Work out the finished part from the listing and answer in its coordinate system (mm). A direction names the side the tool comes from. Round coordinates to 2 decimals unless told otherwise and drop trailing zeros. Write each loop counter-clockwise with the first axis right and the second up, starting at its lowest first coordinate (ties: lowest second). Pieces come first, ordered by that corner, then holes. Notation, with made-up numbers: M 47.25,-28 L 83.25,-28 A26 ccw 83.25,-12 Z; hole C 51,10.25 d11. An arc over 180 degrees is marked long. Answer in a Markdown table with one row per item.
```python
from build123d import *

# Parameters (mm, degrees)
F0_W      = 91.4067700505
F0_H      = 67.4502924085
F1_DEPTH  = 12.7
F3_DEPTH  = 25.4
F4_W      = 51.4017706737
F4_H      = 34.0803191066
F5_DEPTH  = 7.62
F6_W      = 21.1654342711
F6_H      = 34.0803191066
F7_DEPTH  = 25.4
F8_W      = 23.9177821204
F8_H      = 19.4233638573
F9_DEPTH  = 25.4
F10_W     = 14.652994927
F10_H     = 34.0803191066
F11_DEPTH = 7.62
F13_DEPTH = 10.16
F15_DEPTH = 25.4
F17_DEPTH = 25.4
F18_DEPTH = 10.16
F19_W     = 15.5833414756
F19_H     = 10.1625369862
F20_DEPTH = 10.16
F23_D     = 8.89


with BuildPart() as f1:
    # F0 (on Top) → F1 (new body)
    with BuildSketch(Plane.XY):
        with Locations((-3.4888088703, -14.8855820298)):
            Rectangle(F0_W, F0_H)
    extrude(amount=F1_DEPTH)

    # F2 (on face) → F3 (cut)
    with BuildSketch(Plane.XY.offset(12.7)):
        Polygon((-49.1921938956, 18.8395641744), (-49.1921938956, 0), (-15.6996361911, 18.8395641744), align=None)
        Polygon((-15.6996361911, -48.6107282341), (-49.1921938956, -23.0261329561), (-49.1921938956, -48.6107282341), align=None)
    extrude(amount=-F3_DEPTH, mode=Mode.SUBTRACT)

    # F4 (on face) → F5 (join)
    with BuildSketch(Plane.XY.offset(12.7)):
        with Locations((16.5136908181, -17.0401595533)):
            Rectangle(F4_W, F4_H)
    extrude(amount=F5_DEPTH)

    # F6 (on face) → F7 (join)
    with BuildSketch(Plane.XY.offset(20.32)):
        with Locations((31.6318590194, -17.0401595533)):
            Rectangle(F6_W, F6_H)
    extrude(amount=F7_DEPTH)

    # F8 (on face) → F9 (cut)
    with BuildSketch(Plane(origin=(21.0491418839, 0, 0), x_dir=(0, -1, 0), z_dir=(-1, 0, 0))):
        with Locations((22.1214280464, 30.0316819286)):
            Rectangle(F8_W, F8_H)
    extrude(amount=-F9_DEPTH, mode=Mode.SUBTRACT)

    # F10 (on face) → F11 (cut)
    with BuildSketch(Plane.XY.offset(20.32)):
        with Locations((-1.8606970552, -17.0401595533)):
            Rectangle(F10_W, F10_H)
    extrude(amount=-F11_DEPTH, mode=Mode.SUBTRACT)

    # F12 (on face) → F13 (join)
    with BuildSketch(Plane.XY.offset(20.32)):
        Polygon((21.0491418839, 0), (5.4658004083, 0), (5.4658004083, -13.4125072509), (21.0491418839, -13.4125072509), (21.0491418839, -10.1625369862), align=None)
    extrude(amount=F13_DEPTH)

    # F14 (on face) → F15 (cut)
    with BuildSketch(Plane.XY.offset(12.7)):
        Polygon((-28.525055022, -38.8135323032), (-28.525055022, 11.6252659037), (-49.1921938956, 0), (-49.1921938956, -23.0261329561), align=None)
    extrude(amount=-F15_DEPTH, mode=Mode.SUBTRACT)

    # F16 (on face) → F17 (cut)
    with BuildSketch(Plane.XY.offset(12.7)):
        Polygon((-28.525055022, 11.6252659037), (-28.525055022, -3.0236337334), (0, 18.8395641744), (-15.6996361911, 18.8395641744), align=None)
        Polygon((0, -48.6107282341), (-28.525055022, -28.1430520117), (-28.525055022, -38.8135323032), (-15.6996361911, -48.6107282341), align=None)
    extrude(amount=-F17_DEPTH, mode=Mode.SUBTRACT)

    # F18 (cut): a face of the model
    f18_faces = [f1.faces().sort_by_distance(p)[0] for p in [
        (13.2574711461, -6.7062536255, 30.48),
    ]]
    extrude(f18_faces, amount=-F18_DEPTH, mode=Mode.SUBTRACT)

    # F19 (on face) → F20 (join)
    with BuildSketch(Plane.XY.offset(20.32)):
        with Locations((13.2574711461, -5.0812684931)):
            Rectangle(F19_W, F19_H)
    extrude(amount=F20_DEPTH)

    # F23 (through all)
    with Locations(Plane.XY.offset(12.7)):
        with Locations((26.8638245761, 10.2338371798), (29.4222831726, -41.6331104934)):
            Hole(F23_D / 2)


solid = f1.part
```
1. Given pin 1 (1 mm diameter, centred on x = 24, z = 16, fed in from -Y); pin 2 (9 mm diameter, centred on y = -17, z = 25.5, fed in from -X); pin 3 (3 mm diameter, centred on x = 18, z = 23.5, fed in from +Y); pin 4 (10 mm diameter, centred on x = 26.86, y = 10.23, fed in from +Z), each flat-ended and moving along its own axis, determine where each tip first touches the part or whether it passes through.
Calculated:
| item | result |
|---|---|
| pin 1 | stops at y = -34.08 |
| pin 2 | passes through |
| pin 3 | stops at y = 0 |
| pin 4 | stops at z = 12.7 |
2. Determine the mould class of faces 1 (the flat face through (42.215, -15, 17)), 2 (the flat face through (24, -22, 20.32)), 3 (the flat face through (13, -5, 30.48)), 4 (the flat face through (28, -10.163, 28)) for opening direction Z: released by +Z, released by -Z, zero draft, split by the parting line, or undercut.
Calculated:
| item | result |
|---|---|
| face 1 | zero draft |
| face 2 | undercut |
| face 3 | released by +Z |
| face 4 | undercut |
3. A tool of negligible diameter and unlimited length cuts with its end or side. For faces 5 (the flat face through (24, -34.08, 16)), 6 (the flat face through (28, 0, 25)), 7 (the flat face through (31, -22, 39.743)), 8 (the flat face through (5.466, -13, 19)), from which of +Z, -Z, +X, -X, +Y, -Y can it reach the whole face along a straight path? Write none if from no direction.
Calculated:
| item | result |
|---|---|
| face 5 | +Z, +X, -X, -Y |
| face 6 | +Z, +X, -X, +Y |
| face 7 | +X, -X, -Y |
| face 8 | +Z, -X, +Y, -Y |
4. The part is cut by section B-B (x = 33). Determine the outline of the cut face in (y, z).
Calculated:
| item | result |
|---|---|
| outline | M -48.61,0 L -44.27,0 L -44.27,12.7 L -48.61,12.7 Z; M -39,0 L 18.84,0 L 18.84,12.7 L 0,12.7 L 0,45.72 L -34.08,45.72 L -34.08,39.74 L -10.16,39.74 L -10.16,20.32 L -34.08,20.32 L -34.08,12.7 L -39,12.7 Z |
5. Consider line 1 along Z through (x, y) = (32.5, -34); line 2 along X through (y, z) = (-6.5, 19.5); line 3 along Y through (x, z) = (9, 18.5). Determine where each line is inside the solid, lowest interval first. Write a range as from..to.
Calculated:
| item | result |
|---|---|
| line 1 | z = 0..20.32, 39.74..45.72 |
| line 2 | x = 5.47..42.21 |
| line 3 | y = -34.08..0 |
6. The part is cut by section A-A (y = -24). Determine the outline of the cut face in (x, z), plus the area to 3 significant figures.
Calculated:
| item | result |
|---|---|
| outline | M -28.53,0 L 42.21,0 L 42.21,20.32 L 5.47,20.32 L 5.47,12.7 L -28.53,12.7 Z; M 21.05,39.74 L 42.21,39.74 L 42.21,45.72 L 21.05,45.72 Z |
| area | 1,300 mm² |
7. The part is cut by section D-D (y = -8.5). Determine the outline of the cut face in (x, z).
Calculated:
| item | result |
|---|---|
| outline | M -28.53,0 L 42.21,0 L 42.21,45.72 L 21.05,45.72 L 21.05,30.48 L 5.47,30.48 L 5.47,12.7 L -28.53,12.7 Z |
8. The part is cut by section C-C (z = 9). Determine the outline of the cut face in (x, y) (3 decimals).
Calculated:
| item | result |
|---|---|
| outline | M -28.525,-28.143 L 0,-48.611 L 42.215,-48.611 L 42.215,18.84 L 0,18.84 L -28.525,-3.024 Z; hole C 26.864,10.234 d8.89; hole C 29.422,-41.633 d8.89 |
